Check sheet for the modelled part. Datum: model origin and axes. Units: mm. A direction names the side the tool comes from. Round coordinates to 2 decimals unless told otherwise and drop trailing zeros. Write each loop counter-clockwise with the first axis right and the second up, starting at its lowest first coordinate (ties: lowest second). Pieces come first, ordered by that corner, then holes. Notation, with made-up numbers: (27.5, 59.5) -> (32.5, 59.5) arc R19 ccw to (32.5, 82.5) -> close; hole circle Ø9 at (23.25, -4.5). An arc over 180 degrees is marked (long way). Write item = value, one per line.
from build123d import *

# Parameters (mm, degrees)
BOSS_EXTRUDE1_DEPTH = 9
CIRPATTERN1_COUNT   = 2


# Read off the part's stored shape, not the designer's step: M8x1.0 Tapped Hole1
with BuildPart() as part:
    # Sketch1 → Boss-Extrude1 (new, symmetric)
    with BuildSketch(Plane(origin=(0, 0, 0), x_dir=(1, 0, 0), z_dir=(0, 1, 0))):
        with BuildLine():
            Line((-25.4, 0), (25.4, 0))
            Line((25.4, 0), (25.4, 31.75))
            Line((25.4, 31.75), (-25.4, 31.75))
            Line((-25.4, 31.75), (-25.4, 21.5))
            Line((-25.4, 21.5), (5.4, 21.5))
            ThreePointArc((5.4, 21.5), (9.4, 17.5), (5.4, 13.5))
            Line((5.4, 13.5), (-25.4, 13.5))
            Line((-25.4, 13.5), (-25.4, 0))
        make_face()
    boss_extrude1 = extrude(amount=BOSS_EXTRUDE1_DEPTH, both=True)

    # M8x1.0 Tapped Hole1 outline → M8x1.0 Tapped Hole1 (revolve, cut)
    with BuildSketch(Plane.XZ):
        Polygon((4, -21.5), (0, -21.5), (0, -31.75), (4, -31.75), (3.5, -31.25), (3.5, -22), align=None)
    m8x1_0_tapped_hole1 = revolve(axis=Axis((0, 0, 0), (0, 0, 1)), mode=Mode.SUBTRACT)

    # CirPattern1: Boss-Extrude1, M8x1.0 Tapped Hole1 ×2 about axis
    cirpattern1_axis = Axis((0, 0, 0), (0, 1, 0))
    add([boss_extrude1.rotate(cirpattern1_axis, i * 360 / CIRPATTERN1_COUNT) for i in range(1, CIRPATTERN1_COUNT)])
    add([m8x1_0_tapped_hole1.rotate(cirpattern1_axis, i * 360 / CIRPATTERN1_COUNT) for i in range(1, CIRPATTERN1_COUNT)], mode=Mode.SUBTRACT)

    # Sketch5 → Revolve1 (revolve)
    with BuildSketch(Plane(origin=(0, 0, 0), x_dir=(1, 0, 0), z_dir=(0, 1, 0)), mode=Mode.PRIVATE) as revolve1_sk:
        Polygon((25.4, 0), (51.171225178, 0), (51.171225178, 2), (38.15, 2), (33.4, 6.75), (25.4, 6.75), align=None)
    revolve(revolve1_sk.sketch.rotate(Axis((-80.9, 0, 0), (1, 0, 0)), 180), axis=Axis((-80.9, 0, 0), (1, 0, 0)))


solid = part.part
(1) Sectioned sample at A-A on x = 0. Enter the section's corners in (y, z), then the cut area to 4 significant figures.
Worked answers:
outline = (-9, -31.75) -> (-4, -31.75) -> (-3.5, -31.25) -> (-3.5, -22) -> (-4, -21.5) -> (-9, -21.5) -> close; (-9, -13.5) -> (9, -13.5) -> (9, 13.5) -> (-9, 13.5) -> close; (-9, 21.5) -> (-4, 21.5) -> (-3.5, 22) -> (-3.5, 31.25) -> (-4, 31.75) -> (-9, 31.75) -> close; (3.5, -31.25) -> (4, -31.75) -> (9, -31.75) -> (9, -21.5) -> (4, -21.5) -> (3.5, -22) -> close; (3.5, 22) -> (4, 21.5) -> (9, 21.5) -> (9, 31.75) -> (4, 31.75) -> (3.5, 31.25) -> close
area = 710.5 mm²
(2) Sectioned sample at D-D on y = 0. Count the separate pieces of the cut face and the enclosed holes in it, then the cut area to 3 significant figures.
Worked answers:
separate_pieces = 3
enclosed_holes = 0
area = 2,740 mm²
(3) Release check for a two-part mould opening along Y. For faces 4 (the cylindrical face through (29.34, 6.59, -1.46)), 5 (the flat face through (-25.4, 0, -27)), 6 (the cylindrical face through (3.233, -1.341, -26.56)), 7 (the cylindrical face through (-3.233, -1.341, 26.56)) record: pulls with the +Y half, pulls with the -Y half, needs draft (parallel to the pull), parting line crosses it, or undercut.
Worked answers:
face_4 = parting line crosses it
face_5 = needs draft
face_6 = undercut
face_7 = undercut
(4) Access from +Z, -Z, +X, -X, +Y, -Y to the whole of each face (thin tool, end or side, straight path). Record for faces 1 (the flat face through (-10, 0, -13.5)), 2 (the flat face through (-5, 0, -31.75)), 3 (the flat face through (10, 0, 13.5)).
Worked answers:
face_1 = -X, +Y, -Y
face_2 = -Z, +X, -X, +Y, -Y
face_3 = +X, +Y, -Y
(5) Sectioned sample at B-B on z = 0. Enter the section's corners in (x, y), then the cut area to 3 significant figures.
Worked answers:
outline = (-25.4, -9) -> (25.4, -9) -> (25.4, -6.75) -> (33.4, -6.75) -> (38.15, -2) -> (51.17, -2) -> (51.17, 2) -> (38.15, 2) -> (33.4, 6.75) -> (25.4, 6.75) -> (25.4, 9) -> (-25.4, 9) -> close
area = 1,120 mm²
(6) Go/stop test with flat-tipped pins: P1, Ø10, axis at x = 42, z = 0, coming from the -Y side; P2, Ø5, axis at x = 41.5, y = 2.5, coming from the +Z side; P3, Ø5.5, axis at x = 2.5, y = 0, coming from the +Z side; P4, Ø4, axis at x = 0, y = 0, coming from the +Z side. Record where each tip stops, or that it passes through.
Worked answers:
P1 = -3.15
P2 = 2
P3 = 31.75
P4 = 13.5
(7) Sectioned sample at C-C on x = 17. Enter the section's corners in (y, z).
Worked answers:
outline = (-9, -31.75) -> (9, -31.75) -> (9, 13.5) -> (-9, 13.5) -> close; (-9, 21.5) -> (9, 21.5) -> (9, 31.75) -> (-9, 31.75) -> close
(8) Material ranges on L1, parallel to Z at x = -5, y = 5.25; L2, parallel to Y at x = 0, z = -25; L3, parallel to Z at x = 24, y = -2.75, recorded low to high. Write a range as [from, to].
Worked answers:
L1 = [-31.75, -21.5], [-13.5, 13.5], [21.5, 31.75]
L2 = [-9, -3.5], [3.5, 9]
L3 = [-31.75, 13.5], [21.5, 31.75]
